Geometry: final body of the model. Coordinates: model frame, mm. Face numbers are marked on the shaded views. Give positions to 0.01 mm unless a question says otherwise; leave off trailing zeros. Order: outer loops, then holes, each group sorted by start corner. A loop starts at its lowest first (then second) coordinate and runs counter-clockwise, first axis right, second up. Notation, with made-up numbers: (-16, 57.25) -> (-4, 57.25) arc R18 ccw to (-4, 65.25) -> close; hole circle Ø3 at (22, 11.5). An arc over 180 degrees is marked (long way). One line per item, written item: value. Start each with the question number.
```python
from build123d import *

# Parameters (mm, degrees)
SKETCH1_R           = 75
BASE_PLATE_DEPTH    = 15
SKETCH2_R           = 4.5
DRIVE_HOLES_DEPTH   = 10
CHAMFER1_SIZE       = 1
BASE_START          = 45
BASE_FIN_DEPTH      = 5
BASE_START_2        = 85
BASE_FIN_2_DEPTH    = 5
CUT_EXTRUDE1_REACH  = 122
CUT_EXTRUDE2_REACH  = 122
SKETCH7_R           = 1.75
BOSS_EXTRUDE1_DEPTH = 5.6
SKETCH9_R           = 1.75
CUT_EXTRUDE3_DEPTH  = 5.6
SKETCH10_W          = 4.6
SKETCH10_H          = 2.5
SKETCH10_W_2        = 6
CUT_EXTRUDE4_DEPTH  = 5.6
CUT_EXTRUDE5_DEPTH  = 2.6
BOSS_EXTRUDE2_DEPTH = 1.38
FILLET1_R           = 2
FILLET2_R           = 2
CUT_EXTRUDE6_REACH  = 37
SKETCH13_R          = 12.5


with BuildPart() as part:
    # Sketch1 → Base Plate (new body)
    with BuildSketch(Plane.XY):
        Circle(SKETCH1_R)
    extrude(amount=BASE_PLATE_DEPTH)

    # Sketch2 → Drive Holes (cut)
    with BuildSketch(Plane(origin=(0, 0, 0), x_dir=(-1, 0, 0), z_dir=(0, 0, -1))):
        with Locations((0, -25)):
            Circle(SKETCH2_R)
        with Locations((-23.776412907, -7.725424859)):
            Circle(SKETCH2_R)
        with Locations((-14.694631307, 20.225424859)):
            Circle(SKETCH2_R)
        with Locations((14.694631307, 20.225424859)):
            Circle(SKETCH2_R)
        with Locations((23.776412907, -7.725424859)):
            Circle(SKETCH2_R)
    extrude(amount=-DRIVE_HOLES_DEPTH, mode=Mode.SUBTRACT)

    # Chamfer1
    chamfer1_edges = [part.edges().sort_by_distance(p)[0] for p in [
        (28.276412907, -7.725424859, 0),
        (19.194631307, 20.225424859, 0),
        (-10.194631307, 20.225424859, 0),
        (-19.276412907, -7.725424859, 0),
        (4.5, -25, 0),
    ]]
    chamfer(chamfer1_edges, length=CHAMFER1_SIZE)

    # Sketch4 → Base Fin (add)
    with BuildSketch(Plane(origin=(0, 0, 0), x_dir=(0, 0, -1), z_dir=(1, 0, 0)).offset(BASE_START)):
        with BuildLine():
            Line((-15, 50), (-65.791986374, 16.233382914))
            ThreePointArc((-65.791986374, 16.233382914), (-74.493324261, 0), (-65.791986374, -16.233382914))
            Line((-65.791986374, -16.233382914), (-15, -50))
            Line((-15, -50), (-15, 50))
        make_face()
    extrude(amount=-BASE_FIN_DEPTH)

    # Sketch5 → Base Fin 2 (add)
    with BuildSketch(Plane.ZY.offset(-40).offset(BASE_START_2)):
        with BuildLine():
            Line((15, 50), (15, -50))
            Line((15, -50), (65.791986374, -16.233382914))
            ThreePointArc((65.791986374, -16.233382914), (74.493324261, 0), (65.791986374, 16.233382914))
            Line((65.791986374, 16.233382914), (15, 50))
        make_face()
    extrude(amount=-BASE_FIN_2_DEPTH)

    # Sketch6 → Cut-Extrude1 (cut, up to next)
    with BuildSketch(Plane.ZY.offset(45), mode=Mode.PRIVATE) as cut_extrude1_sk1:
        with BuildLine():
            Line((64, 8.832492425), (64, -9.567507575))
            ThreePointArc((64, -9.567507575), (63.487436867, -10.804944442), (62.25, -11.317507575))
            Line((62.25, -11.317507575), (24.05, -11.317507575))
            ThreePointArc((24.05, -11.317507575), (22.812563133, -10.804944442), (22.3, -9.567507575))
            Line((22.3, -9.567507575), (22.3, 8.832492425))
            ThreePointArc((22.3, 8.832492425), (22.812563133, 10.069929292), (24.05, 10.582492425))
            Line((24.05, 10.582492425), (62.25, 10.582492425))
            ThreePointArc((62.25, 10.582492425), (63.487436867, 10.069929292), (64, 8.832492425))
        make_face()
    cut_extrude1_tool1 = extrude(cut_extrude1_sk1.sketch, amount=-CUT_EXTRUDE1_REACH, mode=Mode.PRIVATE) & part.part
    add(cut_extrude1_tool1.solids().sort_by_distance((-45, -0.367508, 43.15))[0], mode=Mode.SUBTRACT)

    # Sketch7 → Cut-Extrude2 (cut, up to next)
    with BuildSketch(Plane.ZY.offset(45), mode=Mode.PRIVATE) as cut_extrude2_sk1:
        with Locations((18.35, 4.632492425)):
            Circle(SKETCH7_R)
    cut_extrude2_tool1 = extrude(cut_extrude2_sk1.sketch, amount=-CUT_EXTRUDE2_REACH, mode=Mode.PRIVATE) & part.part
    add(cut_extrude2_tool1.solids().sort_by_distance((-45, 4.632492, 18.35))[0], mode=Mode.SUBTRACT)
    # Sketch7 → Cut-Extrude2 (cut, up to next)
    with BuildSketch(Plane.ZY.offset(45), mode=Mode.PRIVATE) as cut_extrude2_sk2:
        with Locations((18.35, -5.367507575)):
            Circle(SKETCH7_R)
    cut_extrude2_tool2 = extrude(cut_extrude2_sk2.sketch, amount=-CUT_EXTRUDE2_REACH, mode=Mode.PRIVATE) & part.part
    add(cut_extrude2_tool2.solids().sort_by_distance((-45, -5.367508, 18.35))[0], mode=Mode.SUBTRACT)
    # Sketch7 → Cut-Extrude2 (cut, up to next)
    with BuildSketch(Plane.ZY.offset(45), mode=Mode.PRIVATE) as cut_extrude2_sk3:
        with Locations((67.95, -5.367507575)):
            Circle(SKETCH7_R)
    cut_extrude2_tool3 = extrude(cut_extrude2_sk3.sketch, amount=-CUT_EXTRUDE2_REACH, mode=Mode.PRIVATE) & part.part
    add(cut_extrude2_tool3.solids().sort_by_distance((-45, -5.367508, 67.95))[0], mode=Mode.SUBTRACT)
    # Sketch7 → Cut-Extrude2 (cut, up to next)
    with BuildSketch(Plane.ZY.offset(45), mode=Mode.PRIVATE) as cut_extrude2_sk4:
        with Locations((67.95, 4.632492425)):
            Circle(SKETCH7_R)
    cut_extrude2_tool4 = extrude(cut_extrude2_sk4.sketch, amount=-CUT_EXTRUDE2_REACH, mode=Mode.PRIVATE) & part.part
    add(cut_extrude2_tool4.solids().sort_by_distance((-45, 4.632492, 67.95))[0], mode=Mode.SUBTRACT)

    # Sketch8 → Boss-Extrude1 (add)
    with BuildSketch(Plane.ZY.offset(45)):
        with BuildLine():
            Line((70.95, 4.632492425), (70.95, -5.367507575))
            ThreePointArc((70.95, -5.367507575), (67.95, -8.367507575), (64.95, -5.367507575))
            Line((64.95, -5.367507575), (64.95, 4.632492425))
            ThreePointArc((64.95, 4.632492425), (67.95, 7.632492425), (70.95, 4.632492425))
        make_face()
        with BuildLine():
            Line((15, 7.632492425), (15, 0))
            Line((15, 0), (15, -8.367507575))
            Line((15, -8.367507575), (18.35, -8.367507575))
            ThreePointArc((18.35, -8.367507575), (20.471320344, -7.488827919), (21.35, -5.367507575))
            Line((21.35, -5.367507575), (21.35, 4.632492425))
            ThreePointArc((21.35, 4.632492425), (20.471320344, 6.753812769), (18.35, 7.632492425))
            Line((18.35, 7.632492425), (15, 7.632492425))
        make_face()
    extrude(amount=BOSS_EXTRUDE1_DEPTH)

    # Sketch9 → Cut-Extrude3 (cut)
    with BuildSketch(Plane(origin=(-45, 0, 0), x_dir=(0, 0, -1), z_dir=(1, 0, 0))):
        with Locations((-67.95, -5.367507575)):
            Circle(SKETCH9_R)
        with Locations((-67.95, 4.632492425)):
            Circle(SKETCH9_R)
        with Locations((-18.35, -5.367507575)):
            Circle(SKETCH9_R)
        with Locations((-18.35, 4.632492425)):
            Circle(SKETCH9_R)
    extrude(amount=-CUT_EXTRUDE3_DEPTH, mode=Mode.SUBTRACT)

    # Sketch10 → Cut-Extrude4 (cut)
    with BuildSketch(Plane.ZY.offset(50.6)):
        with Locations((19.05, -0.367507575)):
            Rectangle(SKETCH10_W, SKETCH10_H)
        with Locations((67.95, -0.324654002)):
            Rectangle(SKETCH10_W_2, SKETCH10_H)
    extrude(amount=-CUT_EXTRUDE4_DEPTH, mode=Mode.SUBTRACT)

    # Sketch11 → Cut-Extrude5 (cut)
    with BuildSketch(Plane(origin=(-40, 0, 0), x_dir=(0, 0, -1), z_dir=(1, 0, 0))):
        Polygon((-65.075, -7.027389599), (-65.075, -3.707625551), (-67.95, -2.047743527), (-70.825, -3.707625551), (-70.825, -7.027389599), (-67.95, -8.687271623), align=None)
        Polygon((-65.075, 2.972610401), (-65.075, 6.292374449), (-67.95, 7.952256473), (-70.825, 6.292374449), (-70.825, 2.972610401), (-67.95, 1.312728377), align=None)
        Polygon((-15.475, -7.027389599), (-15.475, -3.707625551), (-18.35, -2.047743527), (-21.225, -3.707625551), (-21.225, -7.027389599), (-18.35, -8.687271623), align=None)
        Polygon((-15.475, 2.972610401), (-15.475, 6.292374449), (-18.35, 7.952256473), (-21.225, 6.292374449), (-21.225, 2.972610401), (-18.35, 1.312728377), align=None)
    extrude(amount=-CUT_EXTRUDE5_DEPTH, mode=Mode.SUBTRACT)

    # Sketch12 → Boss-Extrude2 (add)
    with BuildSketch(Plane(origin=(-40, 0, 0), x_dir=(0, 0, -1), z_dir=(1, 0, 0))):
        with BuildLine():
            Line((-44.572101834, -11.317507575), (-44.572101834, 10.582492425))
            Line((-44.572101834, 10.582492425), (-24.05, 10.582492425))
            ThreePointArc((-24.05, 10.582492425), (-22.812563133, 10.069929292), (-22.3, 8.832492425))
            Line((-22.3, 8.832492425), (-22.3, -9.567507575))
            ThreePointArc((-22.3, -9.567507575), (-22.812563133, -10.804944442), (-24.05, -11.317507575))
            Line((-24.05, -11.317507575), (-44.572101834, -11.317507575))
        make_face()
    extrude(amount=-BOSS_EXTRUDE2_DEPTH)

    # Fillet1
    fillet1_edges = [part.edges().sort_by_distance(p)[0] for p in [
        (-45, -29.183753787, 15),
        (-47.8, -8.367507575, 15),
        (-47.8, 7.632492425, 15),
        (42.5, 50, 15),
        (42.5, -50, 15),
        (45, 0, 15),
        (-42.5, 50, 15),
        (-42.5, -50, 15),
        (-45, 28.816246213, 15),
    ]]
    fillet(fillet1_edges, radius=FILLET1_R)

    # Fillet2
    fillet2_edges = [part.edges().sort_by_distance(p)[0] for p in [
        (-75, 0, 15),
    ]]
    fillet(fillet2_edges, radius=FILLET2_R)

    # Sketch13 → Cut-Extrude6 (cut, up to next)
    with BuildSketch(Plane.ZY.offset(-40), mode=Mode.PRIVATE) as cut_extrude6_sk1:
        with Locations((53.15, -0.367507575)):
            Circle(SKETCH13_R)
    cut_extrude6_tool1 = extrude(cut_extrude6_sk1.sketch, amount=-CUT_EXTRUDE6_REACH, mode=Mode.PRIVATE) & part.part
    add(cut_extrude6_tool1.solids().sort_by_distance((40, -0.367508, 53.15))[0], mode=Mode.SUBTRACT)


solid = part.part
```
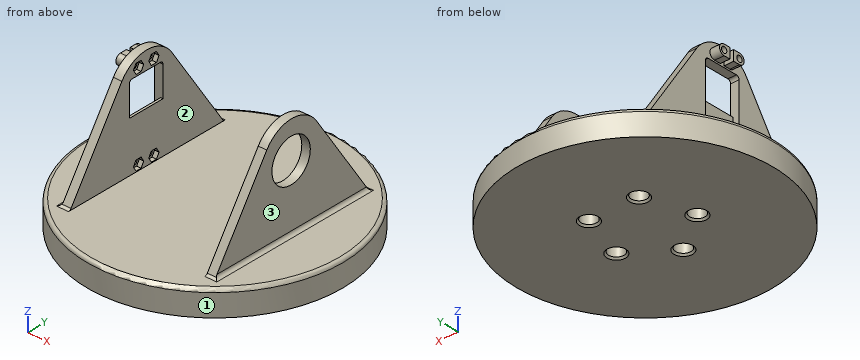
1. Draft query along X for the marked faces 1, 2 and 3. Return one class per face: pulls with the +X half, pulls with the -X half, needs draft (parallel to the pull), parting line crosses it, or undercut.
2. Pin query (flat end, axial travel): P1, Ø6, axis at x = -27.5, y = -42, coming from the +Z side; P2, Ø7, axis at x = 23.5, y = -8.5, coming from the -Z side; P3, Ø12, axis at x = 38, z = 13, coming from the -Y side; P4, Ø1, axis at y = -36.5, z = 39, coming from the -X side. Return the tip coordinate at first contact, or that it passes through.
3. Material intervals for L1, parallel to X at y = -10, z = 38; L2, parallel to Y at x = 0, z = 7; L3, parallel to Y at x = -44.15, z = 18.35, sorted ascending. Write a range as [from, to].
4. Cut plane A-A, the plane z = 53.15. Return loops of the section in (x, y), then the cut area to 3 significant figures.
5. Cut plane B-B, the plane z = 29. Return loops of the section in (x, y), then the cut area to 3 significant figures.
Answers follow:
1. face 1: parting line crosses it
1. face 2: undercut
1. face 3: pulls with the +X half
2. P1: stops at z = 15
2. P2: stops at z = 10
2. P3: stops at y = -67.83
2. P4: passes through
3. L1: x = [-41.38, -40], [40, 45]
3. L2: y = [-75, -29.5], [-20.5, 75]
3. L3: y = [-47.77, -7.12], [-3.62, 2.88], [6.38, 47.77]
4. outline: (-45, -24.64) -> (-40, -24.64) -> (-40, -11.32) -> (-45, -11.32) -> close; (-45, 10.58) -> (-40, 10.58) -> (-40, 24.64) -> (-45, 24.64) -> close; (40, -24.64) -> (45, -24.64) -> (45, -12.87) -> (40, -12.87) -> close; (40, 12.13) -> (45, 12.13) -> (45, 24.64) -> (40, 24.64) -> close
4. area: 258 mm²
5. outline: (-45, -40.69) -> (-40, -40.69) -> (-40, 40.69) -> (-45, 40.69) -> (-45, 10.58) -> (-41.38, 10.58) -> (-41.38, -11.32) -> (-45, -11.32) -> close; (40, -40.69) -> (45, -40.69) -> (45, 40.69) -> (40, 40.69) -> close
5. area: 735 mm²
